Autodesk Inventor part; units mm, degrees
ref_plane "Work Plane2" through (-28.3759, 9.1241, 0) normal (0, 0, 1) x (1, 0, 0)
ref_plane "YZ Plane" through (0, 0, 0) normal (1, 0, 0) x (0, 1, 0)
ref_plane "XZ Plane" through (0, 0, 0) normal (0, 1, 0) x (-1, 0, 0)
sketch "Sketch1" plane through (0, 0, 0) normal (0, 0, 1) x (1, 0, 0)
  line L0 (-28.3759, 9.1241) -> (22.4241, 9.1241)
  line L1 (22.4241, 9.1241) -> (22.4241, -3.5759)
  line L2 (22.4241, -3.5759) -> (-28.3759, -3.5759)
  line L3 (-28.3759, -3.5759) -> (-28.3759, 9.1241)
  point P0 (0, 0)
  dimension "d0" = 50.8
  dimension "d1" = 12.7
extrude "Extrusion1" add sketch "Sketch1" along normal blind 2.54
sketch "Sketch2" plane through (22.4241, -3.5759, 0) normal (1, 0, 0) x (0, 0, -1)
  line L0 (0, 12.7) -> (6.35, 12.7)
  line L1 (6.35, 12.7) -> (6.35, 19.05)
  line L2 (6.35, 19.05) -> (0, 19.05)
  line L3 (0, 19.05) -> (0, 12.7)
  line L4 (0, 0) -> (-2.54, 0)
  line L5 (0, 12.7) -> (-2.54, 12.7)
  line L6 (-1.27, 12.7) -> (-1.27, 0)
  line L7 (-2.54, 12.7) -> (-8.89, 12.7)
  line L8 (-8.89, 12.7) -> (-8.89, 19.05)
  line L9 (-8.89, 19.05) -> (-2.54, 19.05)
  line L10 (-2.54, 19.05) -> (-2.54, 12.7)
  point P0 (0, 3.5759)
  dimension "d4" = 6.35
  dimension "d5" = 6.35
ref_plane "Work Plane2" through (-28.3759, 9.1241, 0) normal (0, 0, 1) x (1, 0, 0)
sketch "Sketch3" plane through (-28.3759, 9.1241, 0) normal (0, 0, 1) x (1, 0, 0)
  line L0 (38.1, 0) -> (31.75, 0)
  line L1 (31.75, 0) -> (31.75, 7.3179)
  line L2 (31.75, 7.3179) -> (38.1, 7.3179)
  line L3 (38.1, 7.3179) -> (38.1, 0)
  line L4 (25.4, 0) -> (19.05, 0)
  line L5 (19.05, 0) -> (19.05, 7.3179)
  line L6 (19.05, 7.3179) -> (25.4, 7.3179)
  line L7 (25.4, 7.3179) -> (25.4, 0)
  line L8 (12.7, 0) -> (6.35, 0)
  line L9 (6.35, 0) -> (6.35, 7.3179)
  line L10 (6.35, 7.3179) -> (12.7, 7.3179)
  line L11 (12.7, 7.3179) -> (12.7, 0)
  line L12 (38.1, 7.3179) -> (50.8, 7.3179)
  line L13 (38.1, 0) -> (38.1, 7.3179)
  line L14 (25.4, 7.3179) -> (31.75, 7.3179)
  line L15 (31.75, 7.3179) -> (31.75, 0)
  line L16 (31.75, 0) -> (25.4, 0)
  line L17 (25.4, 0) -> (25.4, 7.3179)
  line L18 (12.7, 7.3179) -> (19.05, 7.3179)
  line L19 (19.05, 7.3179) -> (19.05, 0)
  line L20 (19.05, 0) -> (12.7, 0)
  line L21 (12.7, 0) -> (12.7, 7.3179)
  line L22 (6.35, 0) -> (0, 0)
  line L23 (0, 0) -> (0, 7.3179)
  line L24 (0, 7.3179) -> (6.35, 7.3179)
  line L25 (6.35, 7.3179) -> (6.35, 0)
  line L26 (50.8, 7.3179) -> (50.8, 0)
  line L27 (50.8, 0) -> (38.1, 0)
  point P0 (28.3759, -9.1241)
extrude "Extrusion4" add sketch "Sketch2" against normal blind 50.8 contours L7 L8 L9 L10
fillet "Fillet2" radius 3.175 3 edges at (-2.9759, 15.4741, 8.89) (-2.9759, 15.4741, 2.54) (-2.9759, 9.1241, 8.89)
extrude "Extrusion5" cut sketch "Sketch3" along normal blind 50.8 contours L3 L12 L26 L27 | L16 L7 L14 L1 | L20 L11 L18 L5 | L22 L23 L24 L9
hole "Hole3" at (9.7241, 12.2991, 5.715) direction (-1, 0, 0) diameter 5.08 end through all
hole "Hole4" at (-16.9459, 2.7741, 2.54) direction (0, 0, -1) diameter 4.9784 end through all
hole "Hole5" at (10.9941, 2.7741, 2.54) direction (0, 0, -1) diameter 4.9784 end through all
hole "Hole6" at (-2.9759, 2.7741, 2.54) direction (0, 0, -1) diameter 4.9784 end through all
sketch "Sketch4" plane through (9.7241, 9.1241, 2.54) normal (0, 0, -1) x (-1, 0, 0)
  line L0 (0, 3.175) -> (0, 0)
  line L1 (6.35, 0) -> (0, 0)
  line L2 (0, 3.175) -> (6.35, 3.175)
  line L3 (6.35, 3.175) -> (6.35, 0)
  line L4 (6.35, 0) -> (0, 0)
  line L5 (0, 0) -> (0, 3.175)
  point P0 (9.7241, -9.1241)
sketch "Sketch5" plane through (-2.9759, 9.1241, 2.54) normal (0, 0, -1) x (-1, 0, 0)
  line L0 (0, 3.175) -> (0, 0)
  line L1 (6.35, 0) -> (0, 0)
  line L2 (0, 3.175) -> (6.35, 3.175)
  line L3 (6.35, 3.175) -> (6.35, 0)
  line L4 (6.35, 0) -> (0, 0)
  line L5 (0, 0) -> (0, 3.175)
  point P0 (-2.9759, -9.1241)
sketch "Sketch6" plane through (-15.6759, 12.2991, 2.54) normal (0, 0, -1) x (-1, 0, 0)
  line L0 (6.35, -3.175) -> (6.35, 0)
  line L1 (0, 0) -> (6.35, 0)
  line L2 (0, 0) -> (6.35, 0)
  line L3 (6.35, 0) -> (6.35, -3.175)
  line L4 (6.35, -3.175) -> (0, -3.175)
  line L5 (0, -3.175) -> (0, 0)
  point P0 (-15.6759, -12.2991)
extrude "Extrusion6" add sketch "Sketch4" along normal blind 2.54
extrude "Extrusion7" add sketch "Sketch5" along normal blind 2.54
extrude "Extrusion8" add sketch "Sketch6" along normal blind 2.54
properties part number "HingeP2"
Input: part model. Units: mm. Frame: model coordinates. A direction names the side the tool comes from. Coordinates: 2 decimals unless noted, no trailing zeros. Write each loop counter-clockwise with the first axis right and the second up, starting at its lowest first coordinate (ties: lowest second). Pieces come first, ordered by that corner, then holes.
1) Section A-A on y = 11.75. Output: boundary loops of the cut face in (x, z).
2) Section B-B on z = 3.75. Output: boundary loops of the cut face in (x, y), and give its area (3 significant figures).
3) Pin query (flat end, axial travel): pin 1 Ø1.9 at (y, z) = (11, 2.5) entering from -X; pin 2 Ø2 at (x, z) = (-24.5, 2) entering from +Y; pin 3 Ø5 at (y, z) = (12, 2.5) entering from +X; pin 4 Ø6 at (x, y) = (-17, 2.5) entering from -Z. Return the tip coordinate at first contact, or that it passes through.
4) Material intervals for line 1 along X through (y, z) = (10, 4); line 2 along X through (y, z) = (4, 0.75); line 3 along Z through (x, y) = (5, 4), sorted ascending.
5) Set-up query: faces 5 (the flat face through (-19, 12.299, 1)), 6 (the flat face through (16, 9.124, 1)), 7 (the flat face through (-6, 9.124, 4)), 8 (the cylindrical face through (-18.895, 14.519, 7.985)), 9 (the flat face through (-13, 9.124, 1)). Return all of +Z, -Z, +X, -X, +Y, -Y with unobstructed straight access to the full face (end or side cutting, diameter ignored); none if empty.
6) Mould query, pull axis Y, two halves, no side actions, for faces 1 (the cylindrical face through (-6.195, 14.569, 3.495)), 2 (the cylindrical face through (13.424, 3.314, 1.252)), 3 (the cylindrical face through (-6.195, 10.029, 7.935)), 4 (the flat face through (-9.326, 10, 4)). Classes: pulls with the +Y half, pulls with the -Y half, needs draft (parallel to the pull), parting line crosses it, or undercut.
7) Section D-D on z = 1. Output: boundary loops of the cut face in (x, y), and give its area (3 significant figures).
8) Section C-C on y = 3.5. Output: boundary loops of the cut face in (x, z), and give its area (3 significant figures).
Check result:
1. outline: (-22.03, 0) - (-15.68, 0) - (-15.68, 3.24) - (-22.03, 3.24) - close; (-22.03, 8.19) - (-15.68, 8.19) - (-15.68, 8.84) - (-22.03, 8.84) - close; (-9.33, 0) - (-2.98, 0) - (-2.98, 3.24) - (-9.33, 3.24) - close; (-9.33, 8.19) - (-2.98, 8.19) - (-2.98, 8.84) - (-9.33, 8.84) - close; (3.37, 0) - (9.72, 0) - (9.72, 3.24) - (3.37, 3.24) - close; (3.37, 8.19) - (9.72, 8.19) - (9.72, 8.84) - (3.37, 8.84) - close
2. outline: (-22.03, 9.12) - (-15.68, 9.12) - (-15.68, 10.69) - (-22.03, 10.69) - close; (-22.03, 13.91) - (-15.68, 13.91) - (-15.68, 14.79) - (-22.03, 14.79) - close; (-9.33, 9.12) - (-2.98, 9.12) - (-2.98, 10.69) - (-9.33, 10.69) - close; (-9.33, 13.91) - (-2.98, 13.91) - (-2.98, 14.79) - (-9.33, 14.79) - close; (3.37, 9.12) - (9.72, 9.12) - (9.72, 10.69) - (3.37, 10.69) - close; (3.37, 13.91) - (9.72, 13.91) - (9.72, 14.79) - (3.37, 14.79) - close
2. area: 46.7 mm2
3. pin 1: stops at x = -22.03
3. pin 2: stops at y = 9.12
3. pin 3: stops at x = 9.72
3. pin 4: stops at z = 0
4. line 1: x = -22.03 to -15.68, -9.33 to -2.98, 3.37 to 9.72
4. line 2: x = -28.38 to -19.11, -14.78 to -5.14, -0.81 to 8.83, 13.16 to 22.42
4. line 3: z = 0 to 2.54
5. face 5: -Z, +X, -X, +Y
5. face 6: +Z, -Z, +X, +Y
5. face 7: +Z, +X, -X, -Y
5. face 8: +Z, +X, -X, +Y
5. face 9: +Z, -Z, +Y
6. face 1: pulls with the +Y half
6. face 2: undercut
6. face 3: pulls with the -Y half
6. face 4: needs draft
7. outline: (-28.38, -3.58) - (22.42, -3.58) - (22.42, 9.12) - (9.72, 9.12) - (9.72, 12.3) - (3.37, 12.3) - (3.37, 9.12) - (-2.98, 9.12) - (-2.98, 12.3) - (-9.33, 12.3) - (-9.33, 9.12) - (-15.68, 9.12) - (-15.68, 12.3) - (-22.03, 12.3) - (-22.03, 9.12) - (-28.38, 9.12) - close; hole circle Ø4.98 at (-16.95, 2.77); hole circle Ø4.98 at (-2.98, 2.77); hole circle Ø4.98 at (10.99, 2.77)
7. area: 647 mm2
8. outline: (-28.38, 0) - (-19.33, 0) - (-19.33, 2.54) - (-28.38, 2.54) - close; (-14.56, 0) - (-5.36, 0) - (-5.36, 2.54) - (-14.56, 2.54) - close; (-0.59, 0) - (8.61, 0) - (8.61, 2.54) - (-0.59, 2.54) - close; (13.38, 0) - (22.42, 0) - (22.42, 2.54) - (13.38, 2.54) - close
8. area: 92.7 mm2
